from build123d import *

# Parameters (mm, degrees)
SKETCH1_W           = 21
SKETCH1_H           = 40
BOSS_EXTRUDE1_DEPTH = 12
SKETCH4_W           = 19
SKETCH4_H           = 10
CUT_EXTRUDE2_DEPTH  = 35
FILLET5_R           = 4
FILLET6_R           = 3
FILLET8_R           = 2


with BuildPart() as part:
    # Sketch1 → Boss-Extrude1 (new body)
    with BuildSketch(Plane(origin=(0, 0, 0), x_dir=(1, 0, 0), z_dir=(0, 1, 0))):
        with Locations((10.5, 20)):
            Rectangle(SKETCH1_W, SKETCH1_H)
    extrude(amount=BOSS_EXTRUDE1_DEPTH)

    # Sketch4 → Cut-Extrude2 (cut)
    with BuildSketch(Plane.XY):
        with Locations((10.5, 6)):
            Rectangle(SKETCH4_W, SKETCH4_H)
    extrude(amount=-CUT_EXTRUDE2_DEPTH, mode=Mode.SUBTRACT)

    # Fillet5
    fillet5_edges = [part.edges().sort_by_distance(p)[0] for p in [
        (0, 6, -40),
        (21, 6, -40),
    ]]
    fillet(fillet5_edges, radius=FILLET5_R)

    # Fillet6
    fillet6_edges = [part.edges().sort_by_distance(p)[0] for p in [
        (21, 12, -18),
        (0, 0, -18),
        (0, 12, -18),
        (10.5, 0, -40),
        (19.828427125, 0, -38.828427125),
        (1.171572875, 0, -38.828427125),
        (10.5, 12, -40),
        (19.828427125, 12, -38.828427125),
        (1.171572875, 12, -38.828427125),
        (21, 0, -18),
    ]]
    fillet(fillet6_edges, radius=FILLET6_R)

    # Fillet8
    fillet8_edges = [part.edges().sort_by_distance(p)[0] for p in [
        (20, 11, -17.5),
        (20, 1, -17.5),
        (1, 1, -17.5),
        (1, 11, -17.5),
    ]]
    fillet(fillet8_edges, radius=FILLET8_R)


solid = part.part
Source: CAD feature listing. Evaluate the final solid. Frame: model axes, mm. A direction names the side the tool comes from. Give positions to 0.01 mm unless a question says otherwise; leave off trailing zeros. Loops run counter-clockwise (first coordinate to the right, second up) from the corner with the lowest first, then second, coordinate; pieces in that order, holes last. Notation, with made-up numbers: (85.25, 58) -> (143.25, 58) arc R35 cw to (143.25, 90) -> close; hole circle Ø11 at (-9.5, 62). An arc over 180 degrees is marked (long way). Use a Markdown table: item, result. Add a question column.
1) Section query C-C, the plane z = -35.5. Return the cut outline in (x, y).
2) Pull-direction query (Y, two-part tool) for faces 3 (the face through (0, 6, -18)), 4 (the face through (10, 1, -17)), 5 (the face through (10, 0, -19)), 6 (the face through (1, 6, -17)); classes: +Y half, -Y half, draft (parallel to the pull), parting line (faces both ways), or undercut.
3) First-contact query: pin 1 (3 mm diameter, centred on x = 9, y = 6, fed in from +Z). Flat tip, straight axial feed; report the tip coordinate or a pass-through.
4) Line query: line 1 along X through (y, z) = (5, -14.5); line 2 along Y through (x, z) = (9.25, -27); line 3 along X through (y, z) = (2.5, -12.5). Output: solid intervals per line, ascending. Write a range as [from, to].
5) Section query D-D, the plane x = 15.75. Return the cut outline in (y, z), then the cut area to 3 significant figures.
6) Section query A-A, the plane z = -5. Return the cut outline in (x, y), then the cut area to 3 significant figures.
7) Reachability of faces 1 (the face through (10, 12, -19)), 2 (the face through (20, 6, -17)) from +Z, -Z, +X, -X, +Y, -Y: full face, straight path, thin tool, end or side. Return the list, or none.
8) Section query B-B, the plane y = 7.5. Return the cut outline in (x, z).
Numbers:
| question | item | result |
|---|---|---|
| 1 | outline | (0, 3) arc R3 ccw to (3, 0) -> (18, 0) arc R3 ccw to (21, 3) -> (21, 9) arc R3 ccw to (18, 12) -> (3, 12) arc R3 ccw to (0, 9) -> close |
| 2 | face 3 | draft |
| 2 | face 4 | undercut |
| 2 | face 5 | -Y half |
| 2 | face 6 | undercut |
| 3 | pin 1 | stops at z = -35 |
| 4 | line 1 | x = [0, 1], [20, 21] |
| 4 | line 2 | y = [0, 1], [11, 12] |
| 4 | line 3 | x = [0.04, 1.06], [19.94, 20.96] |
| 5 | outline | (0, -37) arc R3 ccw to (3, -40) -> (9, -40) arc R3 ccw to (12, -37) -> (12, 0) -> (11, 0) -> (11, -35) -> (1, -35) -> (1, 0) -> (0, 0) -> close |
| 5 | area | 126 mm2 |
| 6 | outline | (0, 3) arc R3 ccw to (3, 0) -> (18, 0) arc R3 ccw to (21, 3) -> (21, 9) arc R3 ccw to (18, 12) -> (3, 12) arc R3 ccw to (0, 9) -> close; hole (1, 3) arc R2 ccw to (3, 1) -> (18, 1) arc R2 ccw to (20, 3) -> (20, 9) arc R2 ccw to (18, 11) -> (3, 11) arc R2 ccw to (1, 9) -> close |
| 6 | area | 57.7 mm2 |
| 7 | face 1 | +Z, -Z, +X, -X, +Y |
| 7 | face 2 | +Z |
| 8 | outline | (0, -36) arc R4 ccw to (4, -40) -> (17, -40) arc R4 ccw to (21, -36) -> (21, 0) -> (20, 0) -> (20, -35) -> (1, -35) -> (1, 0) -> (0, 0) -> close |
